Autodesk Inventor part; units mm, degrees
ref_plane "YZ Plane" through (0, 0, 0) normal (1, 0, 0) x (0, 1, 0)
ref_plane "XZ Plane" through (0, 0, 0) normal (0, 1, 0) x (-1, 0, 0)
ref_plane "XY Plane" through (0, 0, 0) normal (0, 0, 1) x (1, 0, 0)
sketch "Sketch1" plane through (0, 0, 0) normal (0, 0, 1) x (1, 0, 0)
  circle A0 centre (20, 0) radius 2.25
  circle A1 centre (80, 0) radius 2.25
  circle A2 centre (0, 0) radius 85
  line L0 (0, 0) -> (20, 0) construction
  line L1 (20, 0) -> (80, 0) construction
  circle A3 centre (14.1421, 14.1421) radius 2.25
  circle A4 centre (56.5685, 56.5685) radius 2.25
  line L2 (0, 0) -> (14.1421, 14.1421) construction
  line L3 (14.1421, 14.1421) -> (56.5685, 56.5685) construction
  circle A5 centre (0, 20) radius 2.25
  circle A6 centre (0, 80) radius 2.25
  line L4 (0, 0) -> (0, 20) construction
  line L5 (0, 20) -> (0, 80) construction
  circle A7 centre (-14.1421, 14.1421) radius 2.25
  circle A8 centre (-56.5685, 56.5685) radius 2.25
  line L6 (0, 0) -> (-14.1421, 14.1421) construction
  line L7 (-14.1421, 14.1421) -> (-56.5685, 56.5685) construction
  circle A9 centre (-20, 0) radius 2.25
  circle A10 centre (-80, 0) radius 2.25
  line L8 (0, 0) -> (-20, 0) construction
  line L9 (-20, 0) -> (-80, 0) construction
  circle A11 centre (-14.1421, -14.1421) radius 2.25
  circle A12 centre (-56.5685, -56.5685) radius 2.25
  line L10 (0, 0) -> (-14.1421, -14.1421) construction
  line L11 (-14.1421, -14.1421) -> (-56.5685, -56.5685) construction
  circle A13 centre (0, -20) radius 2.25
  circle A14 centre (0, -80) radius 2.25
  line L12 (0, 0) -> (0, -20) construction
  line L13 (0, -20) -> (0, -80) construction
  circle A15 centre (14.1421, -14.1421) radius 2.25
  circle A16 centre (56.5685, -56.5685) radius 2.25
  line L14 (0, 0) -> (14.1421, -14.1421) construction
  line L15 (14.1421, -14.1421) -> (56.5685, -56.5685) construction
  dimension "d0" = 170
  dimension "d1" = 20
  dimension "d2" = 80
  dimension "d3" = 4.5
  dimension "d6" = 360
extrude "Extrusion1" add sketch "Sketch1" against normal blind 0.4 contours A0 | A1 | A2 | A3 | A4 | A5 | A6 | A7 | A8 | A9 | A10 | A11 | A12 | A13 | A14 | A15 | A16
extrude "Extrusion2" add sketch "Sketch1" along normal blind 3 contours A0 | A1 | A3 | A4 | A5 | A6 | A7 | A8 | A9 | A10 | A11 | A12 | A13 | A14 | A15 | A16
chamfer "Chamfer1" distance 0.4 angle 45 1 edges at (-85, 0, -0.4)
properties part number "Deskcap"
Geometry check sheet. Reference: the model listing, model coordinates, mm. A direction names the side the tool comes from. Round coordinates to 2 decimals unless told otherwise and drop trailing zeros. Use a Markdown table: item, result. Add a question column.
(1) Material ranges on line 1 along X through (y, z) = (14.5, 2); line 2 along Z through (x, y) = (-32, 72.5); line 3 along Y through (x, z) = (-21, -0.1), recorded low to high. Write a range as [from, to].
(2) Sectioned sample at A-A, the plane z = 2.4. Count the separate pieces of the cut face and the enclosed holes in it, and give its area (3 significant figures).
(3) Depth check by flat-ended pin: pin 1 (1.5 mm diameter, centred on x = 53.5, z = 1.5, fed in from -Y); pin 2 (1.5 mm diameter, centred on x = 60, y = -24.5, fed in from +Z). Enter the tip coordinate at first touch or a pass-through.
(4) Release check for a two-part mould opening along Y. For faces 3 (the flat face through (-57, -57, 3)), 4 (the cylindrical face through (57.607, -54.572, 1.479)), 5 (the cylindrical face through (-14.63, -11.946, 1.479)), 6 (the cylindrical face through (-77.92, 0.86, 1.48)) record: pulls with the +Y half, pulls with the -Y half, needs draft (parallel to the pull), parting line crosses it, or undercut.
(5) Tool access check on faces 1 (the cylindrical face through (-0.488, 22.196, 1.479)), 2 (the flat face through (-14, -14, 3)). Record the directions out of +Z, -Z, +X, -X, +Y, -Y that give a thin tool (end or side, any length) a straight path to the whole face; none if there is none.
Answers below:
| question | item | result |
|---|---|---|
| 1 | line 1 | [-16.36, -11.92], [11.92, 16.36] |
| 1 | line 2 | [-0.4, 0] |
| 1 | line 3 | [-82.26, 82.26] |
| 2 | separate pieces | 16 |
| 2 | enclosed holes | 0 |
| 2 | area | 254 mm² |
| 3 | pin 1 | through |
| 3 | pin 2 | z = 0 |
| 4 | face 3 | needs draft |
| 4 | face 4 | undercut |
| 4 | face 5 | undercut |
| 4 | face 6 | parting line crosses it |
| 5 | face 1 | +Z |
| 5 | face 2 | +Z, +X, -X, +Y, -Y |
